Model file for the job. Use its own axes, mm. A direction names the side the tool comes from. Coordinates: 2 decimals unless noted, no trailing zeros. Order: outer loops, then holes, each group sorted by start corner. A loop starts at its lowest first (then second) coordinate and runs counter-clockwise, first axis right, second up.
Autodesk Inventor part; units mm, degrees
ref_plane "YZ Plane" through (0, 0, 0) normal (1, 0, 0) x (0, 1, 0)
ref_plane "XZ Plane" through (0, 0, 0) normal (0, 1, 0) x (-1, 0, 0)
ref_plane "XY Plane" through (0, 0, 0) normal (0, 0, 1) x (1, 0, 0)
sketch "Sketch1" plane through (0, 0, 0) normal (0, 1, 0) x (-1, 0, 0)
  line L0 (0, 0) -> (30, 0)
  line L1 (30, 0) -> (30, 45)
  line L2 (30, 45) -> (0, 45)
  line L3 (0, 45) -> (0, 0)
  line L4 (33, 0) -> (-3, 0)
  line L5 (-3, 0) -> (-3, 45)
  line L6 (-3, 45) -> (33, 45)
  line L7 (33, 45) -> (33, 0)
  line L8 (30, 45) -> (0, 45)
  line L9 (0, 45) -> (0, 42)
  line L10 (0, 42) -> (30, 42)
  line L11 (30, 42) -> (30, 45)
  line L12 (24.5, 0) -> (5.5, 0)
  line L13 (5.5, 0) -> (5.5, -3)
  line L14 (5.5, -3) -> (24.5, -3)
  line L15 (24.5, -3) -> (24.5, 0)
  line L16 (24.5, 0) -> (33, 0)
  line L17 (33, 0) -> (33, -3)
  line L18 (33, -3) -> (24.5, -3)
  line L19 (24.5, -3) -> (24.5, 0)
  line L20 (5.5, 0) -> (-3, 0)
  line L21 (-3, 0) -> (-3, -3)
  line L22 (-3, -3) -> (5.5, -3)
  line L23 (5.5, -3) -> (5.5, 0)
  circle A0 centre (28.75, 22.5) radius 1.25
  circle A1 centre (1.25, 22.5) radius 1.25
  circle A2 centre (28.75, 22.5) radius 3.25
  circle A3 centre (1.25, 22.5) radius 3.25
  point P0 (33, 22.5)
  point P1 (33, 22.5)
  point P2 (5.5, 0)
  point P3 (30, 19.5)
  point P4 (0, 19.5)
  point P5 (0, 25.5)
  point P6 (30, 25.5)
  dimension "d0" = 3
  dimension "d1" = 3
  dimension "d2" = 30
  dimension "d3" = 45
  dimension "d4" = 3
  dimension "d5" = 19
  dimension "d6" = 3
  dimension "d7" = 2.5
  dimension "d8" = 2.5
  dimension "d9" = 2
  dimension "d10" = 2
extrude "Extrusion1" add sketch "Sketch1" along normal blind 3
extrude "Extrusion2" add sketch "Sketch1" along normal blind 9.5 contours L4 L5 L6 L3 A3 | L0 L13 L22 L21 L4 | A3 L3 | L3 A3 | L0 L4 L17 L18 L15 | L1 A2 L6 L7 L4 | L3 L2 L1 L10 | A2 L1 | L1 A2
properties part number "dongle shell"
Q1. Cut at C-C, the plane y = 6.75. List the corners of the cut face in (x, z).
Established:
outline: (-33, -3) - (-24.5, -3) - (-24.5, 0) - (-30, 0) - (-30, 19.5) arc R3.25 ccw (long way) to (-30, 25.5) - (-30, 42) - (0, 42) - (0, 25.5) arc R3.25 ccw (long way) to (0, 19.5) - (0, 0) - (-5.5, 0) - (-5.5, -3) - (3, -3) - (3, 45) - (-33, 45) - close; hole circle Ø2.5 at (-28.75, 22.5); hole circle Ø2.5 at (-1.25, 22.5)
Q2. Probe line 1 (Z direction, x = -1.25, y = 7); line 2 (X direction, y = 4, z = 37.5); line 3 (Z direction, x = -27, y = 6.25). List the from-to ranges inside material, lowest first.
Established:
line 1: z = -3 to 0, 19.25 to 21.25, 23.75 to 25.75, 42 to 45
line 2: x = -33 to -30, 0 to 3
line 3: z = -3 to 0, 19.76 to 25.24, 42 to 45
Q3. Cut at D-D, the plane z = 8.5. List the corners of the cut face in (x, y).
Established:
outline: (-33, 0) - (3, 0) - (3, 9.5) - (0, 9.5) - (0, 3) - (-30, 3) - (-30, 9.5) - (-33, 9.5) - close
Q4. Drop a flat-ended pin along its axis: P1, Ø1, axis at x = -21.5, y = 4.5, coming from the -Z side. Give the stop position or say it passes through.
Established:
P1: stops at z = 42
Q5. Which spindle directions (+Z, -Z, +X, -X, +Y, -Y) get a long thin tool onto all of the face, cutting with end or side? Do faces 1 (the face through (-15, 0, 21)), 2 (the face through (-30, 6, 10)), 3 (the face through (-5.5, 6, -1)). Say none if no direction does.
Established:
face 1: +Z, -Z, +X, -X, -Y
face 2: +Y
face 3: -Z, +Y
Q6. Cut at B-B, the plane x = -1.25. List the corners of the cut face in (y, z).
Established:
outline: (0, -3) - (9.5, -3) - (9.5, 0) - (3, 0) - (3, 19.25) - (9.5, 19.25) - (9.5, 21.25) - (0, 21.25) - close; (0, 23.75) - (9.5, 23.75) - (9.5, 25.75) - (3, 25.75) - (3, 42) - (9.5, 42) - (9.5, 45) - (0, 45) - close
Q7. Cut at A-A, the plane z = 22.5. List the corners of the cut face in (x, y).
Established:
outline: (-33, 0) - (-30, 0) - (-30, 9.5) - (-33, 9.5) - close; (-27.5, 0) - (-2.5, 0) - (-2.5, 9.5) - (-4.5, 9.5) - (-4.5, 3) - (-25.5, 3) - (-25.5, 9.5) - (-27.5, 9.5) - close; (0, 0) - (3, 0) - (3, 9.5) - (0, 9.5) - close
Q8. Mould opens along X. For faces 4 (the face through (-33, 5, 21)), 5 (the face through (-15.3, 2.6, -3)), 6 (the face through (-27, 6, 0)) say: pulls with the +X half, pulls with the -X half, needs draft (parallel to the pull), parting line crosses it, or undercut.
Established:
face 4: pulls with the -X half
face 5: needs draft
face 6: undercut
